CAD build for the part. Positions are in the model's coordinates, mm. Face numbers are marked on the shaded views. A direction names the side the tool comes from. Coordinates: 2 decimals unless noted, no trailing zeros. Order: outer loops, then holes, each group sorted by start corner. A loop starts at its lowest first (then second) coordinate and runs counter-clockwise, first axis right, second up. Notation, with made-up numbers: M 46,6 L 57,6 A34 ccw 57,43 Z; hole C -12,59 d11. An arc over 180 degrees is marked long. One line per item, written item: value.
from build123d import *

# Parameters (mm, degrees)
SKETCH_1_R      = 13.5
EXTRUDE_1_DEPTH = 25
CHAMFER_1_SIZE  = 2
SKETCH_2_R      = 2.5
EXTRUDE_2_DEPTH = 15


with BuildPart() as part:
    # 스케치1 → 보스-돌출1 (new body)
    with BuildSketch(Plane.XY):
        Circle(SKETCH_1_R)
    extrude(amount=EXTRUDE_1_DEPTH)

    # 모따기1
    chamfer_1_edges = [part.edges().sort_by_distance(p)[0] for p in [
        (-13.5, 0, 0),
        (-13.5, 0, 25),
    ]]
    chamfer(chamfer_1_edges, length=CHAMFER_1_SIZE)

    # 스케치2 → 보스-돌출2 (add)
    with BuildSketch(Plane(origin=(0, 0, 0), x_dir=(-1, 0, 0), z_dir=(0, 0, -1))):
        Circle(SKETCH_2_R)
    extrude(amount=EXTRUDE_2_DEPTH)


solid = part.part
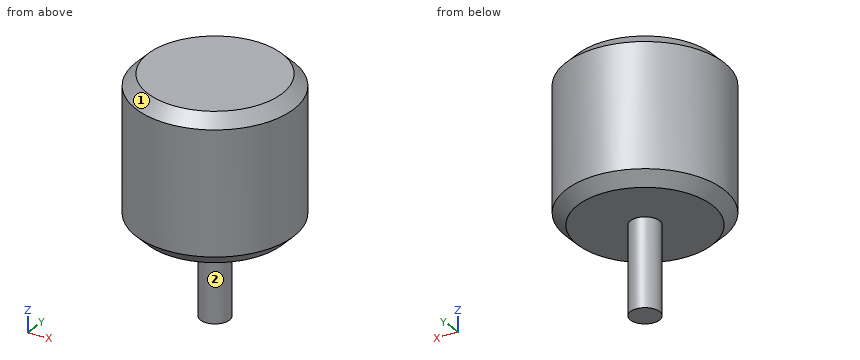
Q1. Pin check, flat tips, straight feed: pin 1 Ø3 at (x, y) = (4, 5.5) entering from -Z; pin 2 Ø12 at (x, z) = (9.5, 12) entering from +Y; pin 3 Ø4 at (y, z) = (2.5, -4.5) entering from +X. Stop position of each tip, or through.
Recorded:
pin 1: stops at z = 0
pin 2: stops at y = 13.04
pin 3: stops at x = 2.45
Q2. Which spindle directions (+Z, -Z, +X, -X, +Y, -Y) get a long thin tool onto all of the face, cutting with end or side? Do the marked faces 1 and 2. Say none if no direction does.
Recorded:
face 1: +Z
face 2: -Z
Q3. Slice it at D-D (z = -9.5). List the corners of the cut face in (x, y).
Recorded:
outline: C 0,0 d5
Q4. Drill centre lines: line 1 along Z through (x, y) = (-7.5, -1); line 2 along Y through (x, z) = (-0.75, 10); line 3 along Y through (x, z) = (-4.5, 4). Where is each one in solid material? Low to high.
Recorded:
line 1: z = 0 to 25
line 2: y = -13.48 to 13.48
line 3: y = -12.73 to 12.73
Q5. Slice it at C-C (z = 15). List the corners of the cut face in (x, y).
Recorded:
outline: C 0,0 d27
Q6. Slice it at A-A (x = 0). List the corners of the cut face in (y, z).
Recorded:
outline: M -13.5,2 L -11.5,0 L -2.5,0 L -2.5,-15 L 2.5,-15 L 2.5,0 L 11.5,0 L 13.5,2 L 13.5,23 L 11.5,25 L -11.5,25 L -13.5,23 Z
